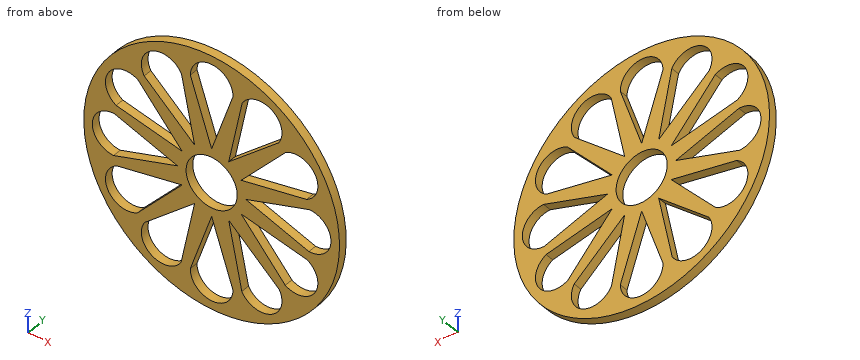
```python
from build123d import *

# Parameters (mm, degrees)
SKETCH1_R         = 30
SKETCH1_R_2       = 6
EXTRUDE1_DEPTH    = 2
EXTRUDE2_DEPTH    = 2
CIRPATTERN1_COUNT = 12


with BuildPart() as part:
    # Sketch1 → Extrude1 (new body)
    with BuildSketch(Plane(origin=(0, 0, 0), x_dir=(1, 0, 0), z_dir=(0, 1, 0))):
        with Locations(Location((0, 0, 0), (0, 0, 270))):
            Circle(SKETCH1_R)
        with Locations(Location((0, 0, 0), (0, 0, 270))):
            Circle(SKETCH1_R_2, mode=Mode.SUBTRACT)
    extrude(amount=EXTRUDE1_DEPTH)

    # Sketch2 → Extrude2 (cut)
    with BuildSketch(Plane(origin=(0, 2, 0), x_dir=(1, 0, 0), z_dir=(0, 1, 0))):
        with BuildLine():
            Line((-5, 22.825230384), (0, 8))
            Line((0, 8), (5.003053509, 23))
            ThreePointArc((5.003053509, 23), (-0.087398144, 28.002290074), (-5, 22.825230384))
        make_face()
    extrude2 = extrude(amount=-EXTRUDE2_DEPTH, mode=Mode.SUBTRACT)

    # CirPattern1: Extrude2 ×12 about axis
    cirpattern1_axis = Axis((0, 0, 0), (0, 1, 0))
    for i in range(1, CIRPATTERN1_COUNT):
        add(extrude2.rotate(cirpattern1_axis, i * 360 / CIRPATTERN1_COUNT), mode=Mode.SUBTRACT)


solid = part.part
```
Source: CAD feature listing. Evaluate the final solid. Frame: model axes, mm. Give positions to 0.01 mm unless a question says otherwise; leave off trailing zeros. Write each loop counter-clockwise with the first axis right and the second up, starting at its lowest first coordinate (ties: lowest second). Pieces come first, ordered by that corner, then holes.
1. Material intervals for line 1 along Z through (x, y) = (9, 1.85); line 2 along Z through (x, y) = (14, 1.95); line 3 along Z through (x, y) = (-20, 1.8), sorted ascending.
2. Section query B-B (z = -11.5). Return the cut outline in (x, y).
3. First-contact query: pin 1 (1 mm diameter, centred on x = -16.5, y = 1.5, fed in from -Z); pin 2 (1.5 mm diameter, centred on x = -7, z = 17, fed in from +Y). Flat tips, straight axial feed; report the tip coordinate or a pass-through.
4. Section query A-A (x = -11.5). Return the cut outline in (y, z).
5. Section query C-C (y = 0.55). Count the separate pieces of the cut face and the enclosed holes in it, then the cut area to 3 significant figures.
Output values:
1. line 1: z = -28.62 to -24.25, -11.36 to -6.35, -4.42 to -0.34, 0.33 to 4.42, 6.34 to 11.33, 24.25 to 28.62
1. line 2: z = -26.53 to -24.25, -15.79 to -12.03, -5.45 to -2.02, 2 to 5.42, 11.98 to 15.73, 24.25 to 26.53
1. line 3: z = -22.36 to -16.5, -6.63 to -4, 4.05 to 6.67, 16.5 to 22.36
2. outline: (-27.71, 0) - (-24.92, 0) - (-24.92, 2) - (-27.71, 2) - close; (-13.58, 0) - (-9.19, 0) - (-9.19, 2) - (-13.58, 2) - close; (-4.93, 0) - (-1.18, 0) - (-1.18, 2) - (-4.93, 2) - close; (1.17, 0) - (4.92, 0) - (4.92, 2) - (1.17, 2) - close; (9.16, 0) - (13.53, 0) - (13.53, 2) - (9.16, 2) - close; (24.92, 0) - (27.71, 0) - (27.71, 2) - (24.92, 2) - close
3. pin 1: stops at z = -25.38
3. pin 2: passes through
4. outline: (0, -27.71) - (2, -27.71) - (2, -24.92) - (0, -24.92) - close; (0, -13.53) - (2, -13.53) - (2, -9.16) - (0, -9.16) - close; (0, -4.92) - (2, -4.92) - (2, -1.17) - (0, -1.17) - close; (0, 1.18) - (2, 1.18) - (2, 4.93) - (0, 4.93) - close; (0, 9.19) - (2, 9.19) - (2, 13.58) - (0, 13.58) - close; (0, 24.92) - (2, 24.92) - (2, 27.71) - (0, 27.71) - close
5. separate pieces: 1
5. enclosed holes: 13
5. area: 1,340 mm2
